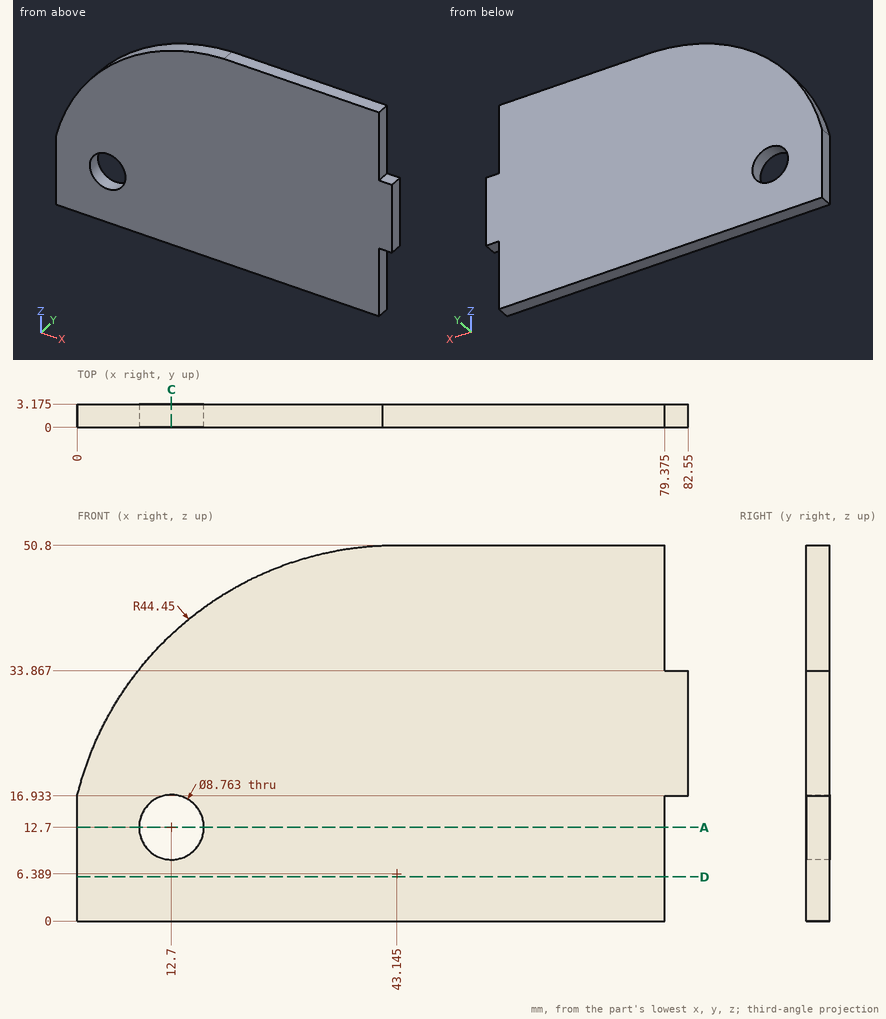
The figure shows three views and two pictorial views of one solid part (mm, origin at its lowest corner). Answer the questions. Coordinates: 2 decimals unless noted, no trailing zeros. Write each loop counter-clockwise with the first axis right and the second up, starting at its lowest first coordinate (ties: lowest second). Pieces come first, ordered by that corner, then holes. Notation, with made-up numbers: (-18.5, -29) -> (0.5, -29) arc R25 ccw to (0.5, -3) -> close; hole circle Ø2 at (-27, -3). An arc over 180 degrees is marked (long way). Return JSON: item names as keys, results as strings.
1. Each of these flat-tipped pins is pushed along its axis until it touches: P1, Ø1, axis at y = 2, z = 39.5, coming from the +X side (3 decimals); P2, Ø1, axis at x = 27.5, z = 18, coming from the -Y side. Where does it stop, or does it pass through?
Found:
{"P1": "x = 79.375", "P2": "y = 0"}
2. A cutting plane is placed at A-A (z = 12.7). Determine the outline of the cut face in (x, y) (1 decimal), and give its area (3 significant figures).
Found:
{"outline": "(0, 0) -> (8.3, 0) -> (8.3, 3.2) -> (0, 3.2) -> close; (17.1, 0) -> (79.4, 0) -> (79.4, 3.2) -> (17.1, 3.2) -> close", "area": "224 mm2"}
3. A cutting plane is placed at C-C (x = 12.7). Determine the outline of the cut face in (y, z) (1 decimal).
Found:
{"outline": "(0, 0) -> (3.2, 0) -> (3.2, 8.3) -> (0, 8.3) -> close; (0, 17.1) -> (3.2, 17.1) -> (3.2, 38.8) -> (0, 38.8) -> close"}
4. Find the intervals of material crossed by line 1 along Z through (x, y) = (12.7, 1) (1 decimal); line 2 along Z through (x, y) = (79.5, 1.2); line 3 along X through (y, z) = (0.5, 9) (1 decimal), in increasing order. Write a range as from..to.
Found:
{"line 1": "0..8.3, 17.1..38.8", "line 2": "16.93..33.87", "line 3": "0..10.4, 15..79.4"}
5. A cutting plane is placed at D-D (z = 6). Determine the outline of the cut face in (x, y) (1 decimal), and give its area (3 significant figures).
Found:
{"outline": "(0, 0) -> (79.4, 0) -> (79.4, 3.2) -> (0, 3.2) -> close", "area": "252 mm2"}
